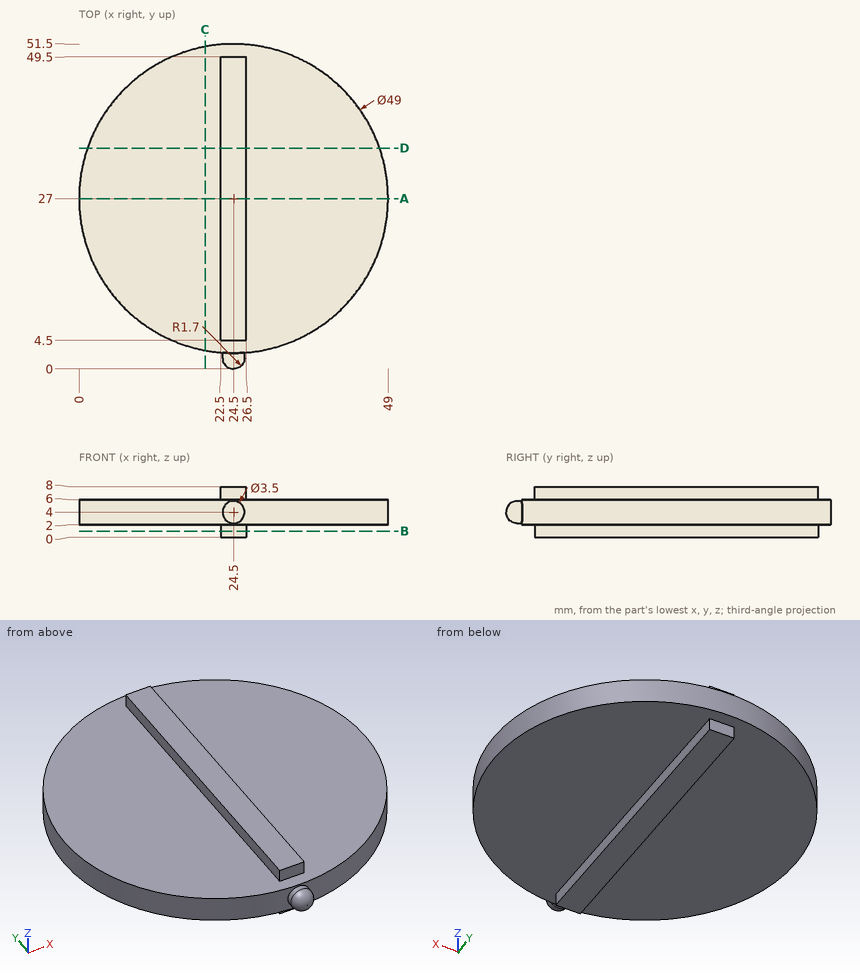
Could you check a few things on this drawing? It's one solid part, dimensions in mm from its lowest x, y, z. Round coordinates to 2 decimals unless told otherwise and drop trailing zeros. Order: outer loops, then holes, each group sorted by start corner. A loop starts at its lowest first (then second) coordinate and runs counter-clockwise, first axis right, second up. Notation, with made-up numbers: M 60,-24.5 L 76,-24.5 A27 cw 76,5.5 Z; hole C 4,-3.5 d4. An arc over 180 degrees is marked long. One line per item, written item: value.
(1) Imagine slicing it at A-A (y = 27). Write out the boundary of the cut face in (x, z).
Ans:
outline: M 0,2 L 22.5,2 L 22.5,0 L 26.5,0 L 26.5,2 L 49,2 L 49,6 L 26.5,6 L 26.5,8 L 22.5,8 L 22.5,6 L 0,6 Z
(2) I need wall thicknesses on line 1 along Z through (x, y) = (30.5, 48.5); line 2 along X through (y, z) = (14.5, 6.25); line 3 along Y through (x, z) = (43.5, 3). Which ranges of each line are inside material? Lowest first, please. Write a range as from..to.
Ans:
line 1: z = 2..6
line 2: x = 22.5..26.5
line 3: y = 11.53..42.47
(3) Imagine slicing it at B-B (z = 1). Write out the boundary of the cut face in (x, y).
Ans:
outline: M 22.5,4.5 L 26.5,4.5 L 26.5,49.5 L 22.5,49.5 Z
(4) Imagine slicing it at C-C (x = 20). Write out the boundary of the cut face in (y, z).
Ans:
outline: M 2.92,2 L 51.08,2 L 51.08,6 L 2.92,6 Z
(5) Imagine slicing it at D-D (y = 35). Write out the boundary of the cut face in (x, z).
Ans:
outline: M 1.34,2 L 22.5,2 L 22.5,0 L 26.5,0 L 26.5,2 L 47.66,2 L 47.66,6 L 26.5,6 L 26.5,8 L 22.5,8 L 22.5,6 L 1.34,6 Z
(6) I'm going to push flat-ended pins straight in: P1, Ø1.6, axis at y = 35.5, z = 7, coming from the -X side; P2, Ø3, axis at x = 16.5, y = 30, coming from the -Z side; P3, Ø1, axis at x = 24, z = 1, coming from the -Y side; P4, Ø10, axis at x = 27.5, y = 31.5, coming from the +Z side. Where does each tip first touch, or does it pass through?
Ans:
P1: stops at x = 22.5
P2: stops at z = 2
P3: stops at y = 4.5
P4: stops at z = 8
